Autodesk Inventor part; units mm, degrees
ref_plane "YZ Plane" through (0, 0, 0) normal (1, 0, 0) x (0, 1, 0)
ref_plane "XZ Plane" through (0, 0, 0) normal (0, 1, 0) x (-1, 0, 0)
ref_plane "XY Plane" through (0, 0, 0) normal (0, 0, 1) x (1, 0, 0)
sketch "Эскиз1" plane through (0, 0, 0) normal (0, 0, 1) x (1, 0, 0)
  circle A0 centre (7.4641, 67.6713) radius 2
  circle A1 centre (7.4641, 364.6713) radius 2
  circle A2 centre (-351.5359, 364.6713) radius 2
  circle A3 centre (-351.5359, 67.6713) radius 2
  line L0 (-359.0359, 370.6713) -> (14.9641, 370.6713)
  line L1 (14.9641, 370.6713) -> (14.9641, 53.6713)
  line L2 (14.9641, 53.6713) -> (-359.0359, 53.6713)
  line L3 (-359.0359, 53.6713) -> (-359.0359, 370.6713)
  line L4 (-359.0359, 370.6713) -> (-367.0359, 370.6713)
  line L5 (-367.0359, 370.6713) -> (-367.0359, 53.6713)
  line L6 (-367.0359, 53.6713) -> (-359.0359, 53.6713)
  line L7 (-359.0359, 53.6713) -> (-359.0359, 370.6713)
  line L8 (14.9641, 370.6713) -> (22.9641, 370.6713)
  line L9 (22.9641, 370.6713) -> (22.9641, 53.6713)
  line L10 (22.9641, 53.6713) -> (14.9641, 53.6713)
  line L11 (14.9641, 53.6713) -> (14.9641, 370.6713)
  dimension "d4" = 374
  dimension "d6" = 317
  dimension "d7" = 14
  dimension "d40" = 7.5
  dimension "d41" = 297
  dimension "d42" = 7.5
  dimension "d43" = 7.5
  dimension "d44" = 297
  dimension "d45" = 6
  dimension "d46" = 359
  dimension "d47" = 14
  dimension "d48" = 359
  dimension "d66" = 8
  dimension "d67" = 8
  dimension "d68" = 390
  dimension "d92" = 4
  dimension "d93" = 4
  dimension "d94" = 4
  dimension "d95" = 4
extrude "Выдавливание1" add sketch "Эскиз1" along normal blind 4
sketch "Эскиз3" plane through (0, 0, 4) normal (0, 0, 1) x (1, 0, 0)
  circle A0 centre (7.4641, 319.6713) radius 5
  circle A1 centre (7.4641, 282.6713) radius 5
  circle A2 centre (-351.5359, 254.6713) radius 2
  point P0 (0, 0)
  dimension "d96" = 10
  dimension "d97" = 10
sketch "Эскиз4" plane through (0, 0, 4) normal (0, 0, 1) x (1, 0, 0)
  circle A0 centre (-171.5359, 372.6713) radius 1.5
  line L0 (-182.5359, 370.6713) -> (-179.0359, 378.6713)
  line L1 (-179.0359, 378.6713) -> (-164.0359, 378.6713)
  line L2 (-164.0359, 378.6713) -> (-160.5359, 370.6713)
  line L3 (22.9641, 370.6713) -> (-367.0359, 370.6713)
  line L4 (-171.5359, 372.6713) -> (-171.5359, 378.6713)
  circle A1 centre (-171.5359, 372.6713) radius 1.5
  point P0 (0, 0)
  point P1 (10.9641, 370.6713)
  point P2 (-363.0359, 370.6713)
  dimension "d49" = 8
  dimension "d50" = 22
  dimension "d51" = 15
sketch "Эскиз5" plane through (0, 0, 0) normal (0, 0, -1) x (-1, 0, 0)
  line L0 (-22.9641, 370.6713) -> (367.0359, 370.6713)
  line L1 (-22.9641, 370.6713) -> (367.0359, 370.6713)
  line L2 (367.0359, 370.6713) -> (367.0359, 561.6713)
  line L3 (367.0359, 561.6713) -> (-22.9641, 561.6713)
  line L4 (-22.9641, 561.6713) -> (-22.9641, 370.6713)
  line L5 (367.0359, 370.6713) -> (367.0359, 53.6713)
  line L6 (-22.9641, 53.6713) -> (-22.9641, 370.6713)
  point P0 (0, 0)
  point P1 (363.0359, 370.6713)
  dimension "d69" = 390
  dimension "d70" = 191
extrude "Выдавливание4" add sketch "Эскиз5" against normal blind 4
extrude "Выдавливание5" cut sketch "Эскиз3" against normal blind 4
extrude "Выдавливание6" cut sketch "Эскиз4" against normal blind 5 contours A0
sketch "Эскиз7" plane through (0, 0, 4) normal (0, 0, 1) x (1, 0, 0)
  circle A0 centre (-353.0359, 403.6713) radius 3.75 construction
  circle A1 centre (-351.0359, 376.6713) radius 3.75 construction
  circle A2 centre (8.9641, 403.6713) radius 3.75 construction
  circle A3 centre (6.9641, 376.6713) radius 3.75 construction
  circle A4 centre (8.9641, 403.6713) radius 5
  circle A5 centre (6.9641, 376.6713) radius 5
  circle A6 centre (-353.0359, 403.6713) radius 5
  circle A7 centre (-351.0359, 376.6713) radius 5
  point P0 (0, 0)
  dimension "d71" = 10
  dimension "d72" = 10
  dimension "d73" = 10
  dimension "d74" = 10
extrude "Выдавливание8" cut sketch "Эскиз7" against normal blind 10
sketch "Эскиз8" plane through (0, 0, 4) normal (0, 0, 1) x (1, 0, 0)
  line L0 (-367.0359, 53.6713) -> (-367.0359, 561.6713)
  line L1 (-367.0359, 561.6713) -> (-289.0359, 561.6713)
  line L2 (-289.0359, 561.6713) -> (-289.0359, 565.6713)
  line L3 (-289.0359, 565.6713) -> (-367.0359, 565.6713)
  line L4 (-367.0359, 565.6713) -> (-367.0359, 561.6713)
  line L5 (-367.0359, 561.6713) -> (22.9641, 561.6713)
  line L6 (-288.7359, 565.6713) -> (-211.3359, 565.6713)
  line L7 (-211.3359, 565.6713) -> (-211.3359, 561.6713)
  line L8 (-211.3359, 561.6713) -> (-288.7359, 561.6713)
  line L9 (-288.7359, 561.6713) -> (-288.7359, 565.6713)
  line L10 (-211.0359, 565.6713) -> (-133.0359, 565.6713)
  line L11 (-133.0359, 565.6713) -> (-133.0359, 561.6713)
  line L12 (-133.0359, 561.6713) -> (-211.0359, 561.6713)
  line L13 (-211.0359, 561.6713) -> (-211.0359, 565.6713)
  line L14 (22.9641, 561.6713) -> (-367.0359, 561.6713)
  line L15 (-132.7359, 561.6713) -> (-55.3359, 561.6713)
  line L16 (-55.3359, 561.6713) -> (-55.3359, 565.6713)
  line L17 (-55.3359, 565.6713) -> (-132.7359, 565.6713)
  line L18 (-132.7359, 565.6713) -> (-132.7359, 561.6713)
  line L19 (22.9641, 561.6713) -> (-55.0359, 561.6713)
  line L20 (-55.0359, 561.6713) -> (-55.0359, 565.6713)
  line L21 (-55.0359, 565.6713) -> (22.9641, 565.6713)
  line L22 (22.9641, 565.6713) -> (22.9641, 561.6713)
  point P0 (0, 0)
  dimension "d77" = 78
  dimension "d78" = 4
  dimension "d79" = 4
  dimension "d80" = 0.3
  dimension "d81" = 0.3
  dimension "d82" = 77.4
  dimension "d83" = 78
  dimension "d84" = 0.3
  dimension "d85" = 4
  dimension "d86" = 77.4
  dimension "d87" = 4
  dimension "d88" = 0.3
  dimension "d89" = 78
extrude "Выдавливание9" add sketch "Эскиз8" against normal blind 4 contours L18 L17 L16 L5 | L9 L6 L7 L5
sketch "Эскиз10" plane through (0, 0, 4) normal (0, 0, 1) x (1, 0, 0)
  line L0 (-329.3859, 556.6713) -> (-329.3859, 561.6713)
  line L1 (-330.6859, 556.6713) -> (-329.3859, 556.6713)
  line L2 (-330.6859, 554.2213) -> (-330.6859, 556.6713)
  line L3 (-329.3859, 554.2213) -> (-330.6859, 554.2213)
  line L4 (-326.3859, 553.1713) -> (-329.3859, 553.1713)
  line L5 (-329.3859, 553.1713) -> (-329.3859, 554.2213)
  line L6 (-326.3859, 554.2213) -> (-326.3859, 553.1713)
  line L7 (-325.0859, 554.2213) -> (-326.3859, 554.2213)
  line L8 (-325.0859, 556.6713) -> (-325.0859, 554.2213)
  line L9 (-326.3859, 556.6713) -> (-325.0859, 556.6713)
  line L10 (-326.3859, 561.6713) -> (-326.3859, 556.6713)
  line L11 (-173.5359, 556.6713) -> (-173.5359, 561.6713)
  line L12 (-170.5359, 561.6713) -> (-170.5359, 556.6713)
  line L13 (-174.8359, 556.6713) -> (-173.5359, 556.6713)
  line L14 (-174.8359, 554.2213) -> (-174.8359, 556.6713)
  line L15 (-173.5359, 554.2213) -> (-174.8359, 554.2213)
  line L16 (-173.5359, 553.1713) -> (-173.5359, 554.2213)
  line L17 (-170.5359, 553.1713) -> (-173.5359, 553.1713)
  circle A0 centre (-353.0359, 403.6713) radius 5
  circle A1 centre (8.9641, 403.6713) radius 5
  circle A2 centre (6.9641, 376.6713) radius 5
  circle A3 centre (-351.0359, 376.6713) radius 5
  circle A4 centre (-171.5359, 372.6713) radius 1.5
  circle A5 centre (7.4641, 319.6713) radius 5
  circle A6 centre (-351.5359, 254.6713) radius 2
  circle A7 centre (7.4641, 282.6713) radius 5
  circle A8 centre (-351.5359, 67.6713) radius 2
  circle A9 centre (-351.5359, 364.6713) radius 2
  circle A10 centre (7.4641, 364.6713) radius 2
  circle A11 centre (7.4641, 67.6713) radius 2
  line L18 (-367.0359, 561.6713) -> (-367.0359, 53.6713)
  line L19 (-367.0359, 53.6713) -> (22.9641, 53.6713)
  line L20 (22.9641, 53.6713) -> (22.9641, 561.6713)
  line L21 (22.9641, 561.6713) -> (-55.3359, 561.6713)
  line L22 (-55.3359, 561.6713) -> (-55.3359, 565.6713)
  line L23 (-55.3359, 565.6713) -> (-132.7359, 565.6713)
  line L24 (-132.7359, 565.6713) -> (-132.7359, 561.6713)
  line L25 (-132.7359, 561.6713) -> (-211.3359, 561.6713)
  line L26 (-211.3359, 561.6713) -> (-211.3359, 565.6713)
  line L27 (-211.3359, 565.6713) -> (-288.7359, 565.6713)
  line L28 (-288.7359, 565.6713) -> (-288.7359, 561.6713)
  line L29 (-288.7359, 561.6713) -> (-367.0359, 561.6713)
  line L30 (-169.2359, 554.2213) -> (-170.5359, 554.2213)
  line L31 (-169.2359, 556.6713) -> (-169.2359, 554.2213)
  line L32 (-170.5359, 556.6713) -> (-169.2359, 556.6713)
  line L33 (-170.5359, 554.2213) -> (-170.5359, 553.1713)
  line L34 (-17.6859, 556.6713) -> (-17.6859, 561.6713)
  line L35 (-14.6859, 561.6713) -> (-14.6859, 556.6713)
  line L36 (-14.6859, 556.6713) -> (-13.3859, 556.6713)
  line L37 (-13.3859, 556.6713) -> (-13.3859, 554.2213)
  line L38 (-13.3859, 554.2213) -> (-14.6859, 554.2213)
  line L39 (-14.6859, 554.2213) -> (-14.6859, 553.1713)
  line L40 (-14.6859, 553.1713) -> (-17.6859, 553.1713)
  line L41 (-17.6859, 553.1713) -> (-17.6859, 554.2213)
  line L42 (-17.6859, 554.2213) -> (-18.9859, 554.2213)
  line L43 (-18.9859, 554.2213) -> (-18.9859, 556.6713)
  line L44 (-18.9859, 556.6713) -> (-17.6859, 556.6713)
  line L45 (-17.6859, 561.6713) -> (-14.6859, 561.6713)
  line L46 (-55.3359, 561.6713) -> (22.9641, 561.6713)
  line L47 (-173.5359, 561.6713) -> (-170.5359, 561.6713)
  line L48 (-329.3859, 561.6713) -> (-326.3859, 561.6713)
  line L49 (-288.7359, 561.6713) -> (-367.0359, 561.6713)
  point P0 (0, 0)
  dimension "d100" = 1.3
  dimension "d101" = 1.3
  dimension "d102" = 1.3
  dimension "d103" = 1.3
  dimension "d104" = 1.3
  dimension "d105" = 1.3
  dimension "d106" = 5
  dimension "d107" = 1.3
  dimension "d108" = 2.45
  dimension "d109" = 8.5
  dimension "d110" = 8.5
  dimension "d111" = 8.5
extrude "Выдавливание10" cut sketch "Эскиз10" against normal blind 10 contours L0 L29 L10 L9 L8 L7 L6 L4 L5 L3 L2 L1 | L35 L36 L37 L38 L39 L40 L41 L42 L43 L44 L34 L21 | L25 L12 L32 L31 L30 L33 L17 L16 L15 L14 L13 L11
properties part number "задняя  панель new"
Verification items for the finished model (mm, model axes). Coordinates: 2 decimals unless noted, no trailing zeros. Answer as a JSON object with one key per item and string values.
(1) Mould release check, pull along Y, two halves, no side actions. Record for faces 1 (the flat face through (-169, 313, 0)), 2 (the cylindrical face through (-348.729, 372.235, 2.028)): pulls with the +Y half, pulls with the -Y half, needs draft (parallel to the pull), parting line crosses it, or undercut.
Report:
{"face 1": "needs draft", "face 2": "undercut"}
(2) Thickness scan on line 1 along X through (y, z) = (402, 3.4); line 2 along Y through (x, z) = (-19.5, 1.2). Record the ranges inside material, lowest first.
Report:
{"line 1": "-367.04 to -357.75, -348.32 to 4.25, 13.68 to 22.96", "line 2": "53.67 to 561.67"}
(3) Gauge pin test, flat ends, axial feed: pin 1 Ø1 at (x, z) = (-14.5, 3) entering from +Y; pin 2 Ø1.2 at (y, z) = (563.5, 2) entering from +X; pin 3 Ø0.9 at (x, z) = (-172, 2) entering from +Y. Record the tip position at first contact, or that the pin passes through.
Report:
{"pin 1": "y = 561.67", "pin 2": "x = -55.34", "pin 3": "y = 553.17"}
